Answer from the drawing. Dimensions are ordinates in mm from the lowest x, y and z of the part. A direction names the side the tool comes from. Coordinates: 2 decimals unless noted, no trailing zeros. Write each loop counter-clockwise with the first axis right and the second up, starting at its lowest first coordinate (ties: lowest second). Pieces come first, ordered by that corner, then holes. Notation, with made-up numbers: (12.5, 34) -> (62.5, 34) arc R18 cw to (62.5, 40) -> close; hole circle Ø1 at (24, 1.5). An arc over 180 degrees is marked (long way). One line per item, written item: value. Start each with the question number.
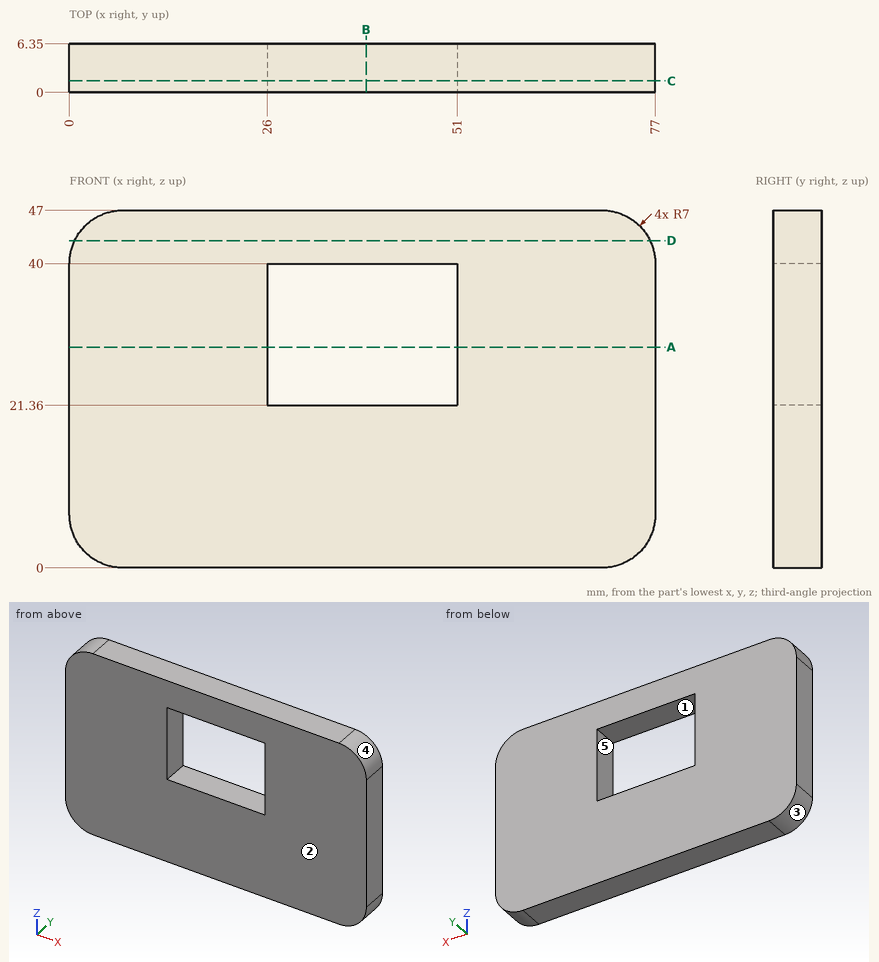
1. For a pull along Z with two mould halves and no side action, classify the marked faces 3, 4 and 5 as +Z half, -Z half, draft (parallel to the pull), parting line (faces both ways), or undercut.
2. A tool of negligible diameter and unlimited length cuts with its end or side. For the marked faces 1 and 2, from which of +Z, -Z, +X, -X, +Y, -Y can it reach the whole face along a straight path? Write none if from no direction.
3. A cutting plane is placed at A-A on z = 29. Give the vertices of the cut face in (x, y), then the cut area to 3 significant figures.
4. A cutting plane is placed at D-D on z = 43. Give the vertices of the cut face in (x, y).
5. Find the intervals of material crossed by probe 1 along X at (y, z) = (5.75, 35); probe 2 along Z at (x, y) = (28.5, 5.5); probe 3 along Z at (x, y) = (70.5, 5.25), in increasing order. Write a range as from..to.
6. A cutting plane is placed at B-B on x = 39. Give the vertices of the cut face in (y, z), then the cut area to 3 significant figures.
7. A cutting plane is placed at C-C on y = 1.5. Give the vertices of the cut face in (x, z).
Derived:
1. face 3: -Z half
1. face 4: +Z half
1. face 5: undercut
2. face 1: +Y, -Y
2. face 2: +Z, -Z, +X, -X, -Y
3. outline: (0, 0) -> (26, 0) -> (26, 6.35) -> (0, 6.35) -> close; (51, 0) -> (77, 0) -> (77, 6.35) -> (51, 6.35) -> close
3. area: 330 mm2
4. outline: (0.68, 0) -> (76.32, 0) -> (76.32, 6.35) -> (0.68, 6.35) -> close
5. probe 1: x = 0..26, 51..77
5. probe 2: z = 0..21.36, 40..47
5. probe 3: z = 0.02..46.98
6. outline: (0, 0) -> (6.35, 0) -> (6.35, 21.36) -> (0, 21.36) -> close; (0, 40) -> (6.35, 40) -> (6.35, 47) -> (0, 47) -> close
6. area: 180 mm2
7. outline: (0, 7) arc R7 ccw to (7, 0) -> (70, 0) arc R7 ccw to (77, 7) -> (77, 40) arc R7 ccw to (70, 47) -> (7, 47) arc R7 ccw to (0, 40) -> close; hole (26, 21.36) -> (51, 21.36) -> (51, 40) -> (26, 40) -> close
